Here's the drawing with two shaded views (mm, measured from the low corner). I have some questions. A direction names the side the tool comes from. Round coordinates to 2 decimals unless told otherwise and drop trailing zeros. Loops run counter-clockwise (first coordinate to the right, second up) from the corner with the lowest first, then second, coordinate; pieces in that order, holes last. Notation, with made-up numbers: M 78,-14.75 L 109,-14.75 A28 cw 109,3.25 Z; hole C 56.5,42 d3. An arc over 180 degrees is marked long. One line per item, written item: value. Start each with the question number.
Q1. Please list where these lines run through material, in increasing order: line 1 along X through (y, z) = (21, 16.5); line 2 along X through (y, z) = (26.9, 10); line 3 along Z through (x, y) = (15, 26.2).
Q2. Imagine slicing it at D-D (z = 16.5). Please give me the cut outline in (x, y), then the cut area to 3 significant figures.
Q3. Imagine slicing it at A-A (x = 35). Please give me the cut outline in (y, z), then the cut area to 3 significant figures.
Q4. Imagine slicing it at B-B (z = 10). Please give me the cut outline in (x, y), then the cut area to 3 significant figures.
Q5. Imagine slicing it at C-C (y = 14.25). Please give me the cut outline in (x, z).
Q6. I'm going to push flat-ended pins straight in: pin 1 Ø10 at (y, z) = (19.5, 11.5) entering from -X; pin 2 Ø3 at (x, z) = (15, 10) entering from -Y; pin 3 Ø5 at (x, z) = (33, 7) entering from -Y. Where does each tip first touch, or does it pass through?
Q7. Which directions (+Z, -Z, +X, -X, +Y, -Y) give clear straight access to the entire face, cutting with the end or side of a thin tool? Please do the marked faces 1 and 2.
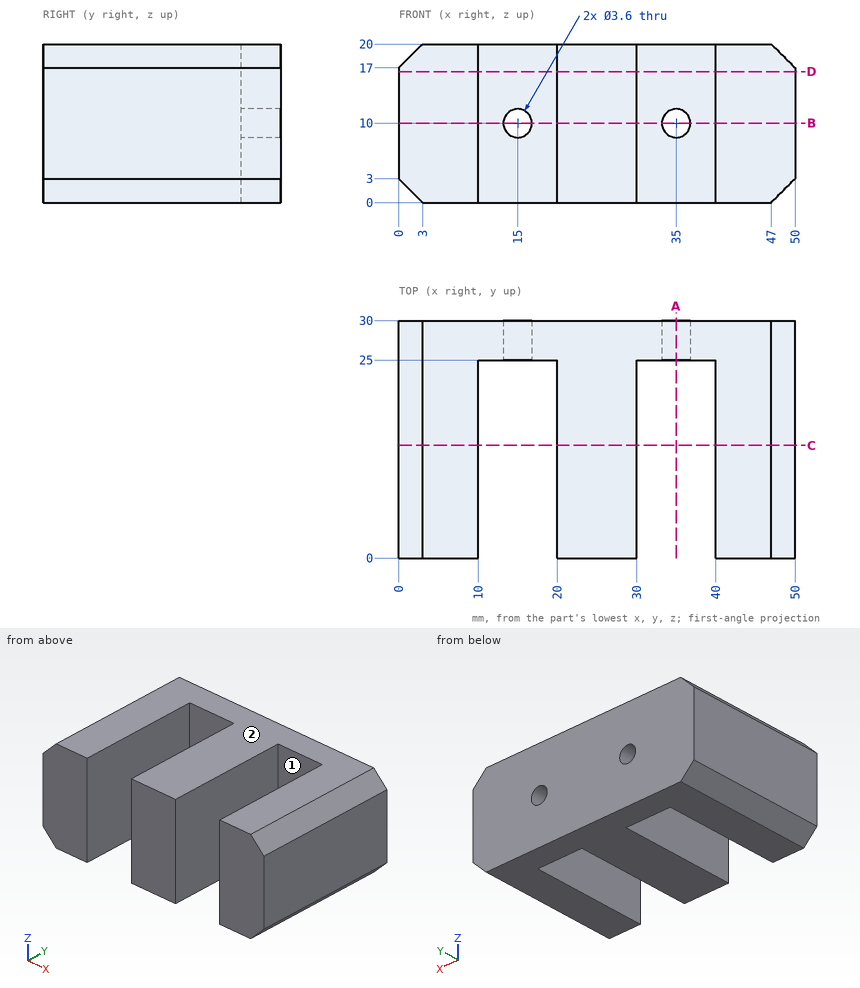
Report:
1. line 1: x = 0 to 10, 20 to 30, 40 to 50
1. line 2: x = 0 to 13.2, 16.8 to 33.2, 36.8 to 50
1. line 3: z = 0 to 8.2, 11.8 to 20
2. outline: M 0,0 L 10,0 L 10,25 L 20,25 L 20,0 L 30,0 L 30,25 L 40,25 L 40,0 L 50,0 L 50,30 L 0,30 Z
2. area: 1,000 mm²
3. outline: M 25,0 L 30,0 L 30,8.2 L 25,8.2 Z; M 25,11.8 L 30,11.8 L 30,20 L 25,20 Z
3. area: 82.0 mm²
4. outline: M 0,0 L 10,0 L 10,25 L 13.2,25 L 13.2,30 L 0,30 Z; M 16.8,25 L 20,25 L 20,0 L 30,0 L 30,25 L 33.2,25 L 33.2,30 L 16.8,30 Z; M 36.8,25 L 40,25 L 40,0 L 50,0 L 50,30 L 36.8,30 Z
4. area: 964 mm²
5. outline: M 0,3 L 3,0 L 10,0 L 10,20 L 3,20 L 0,17 Z; M 20,0 L 30,0 L 30,20 L 20,20 Z; M 40,0 L 47,0 L 50,3 L 50,17 L 47,20 L 40,20 Z
6. pin 1: stops at x = 0
6. pin 2: passes through
6. pin 3: stops at y = 25
7. face 1: +Z, -Z, -Y
7. face 2: +Z, +X, -X, +Y, -Y
